Design review of the part shown in the three views and the two pictorial views. Dimensions are in mm from the part's minimum x, y and z. A direction names the side the tool comes from. Round coordinates to 2 decimals unless told otherwise and drop trailing zeros. Order: outer loops, then holes, each group sorted by start corner. A loop starts at its lowest first (then second) coordinate and runs counter-clockwise, first axis right, second up. Notation, with made-up numbers: (54.5, -11.5) - (70.5, -11.5) arc R24 ccw to (70.5, 24.5) - close; hole circle Ø8 at (1.25, -6.75). An arc over 180 degrees is marked (long way). One line per question, with ' | ' between items. Start each with the question number.
Item 1: Add section B-B on x = 28. State the section outline as (y, z) points, and give its area (3 significant figures).
Item 2: Add section C-C on y = 19. State the section outline as (x, z) points.
Item 3: Tool access review of the marked faces 1, 2 and 3: name each direction out of +Z, -Z, +X, -X, +Y, -Y from which nothing blocks a thin tool from reaching the whole face with its end or side.
Item 4: Add section A-A on z = 64. State the section outline as (x, y) points.
Item 5: For L1, parallel to Y at x = 22, z = 87.5; L2, parallel to Z at x = 46.5, y = 17; L3, parallel to X at y = 29, z = 69.5 (1 decimal), list the stretches that pass through material, from the lowest coordinate up. Write a range as [from, to].
Item 6: Add section D-D on z = 85. State the section outline as (x, y) points.
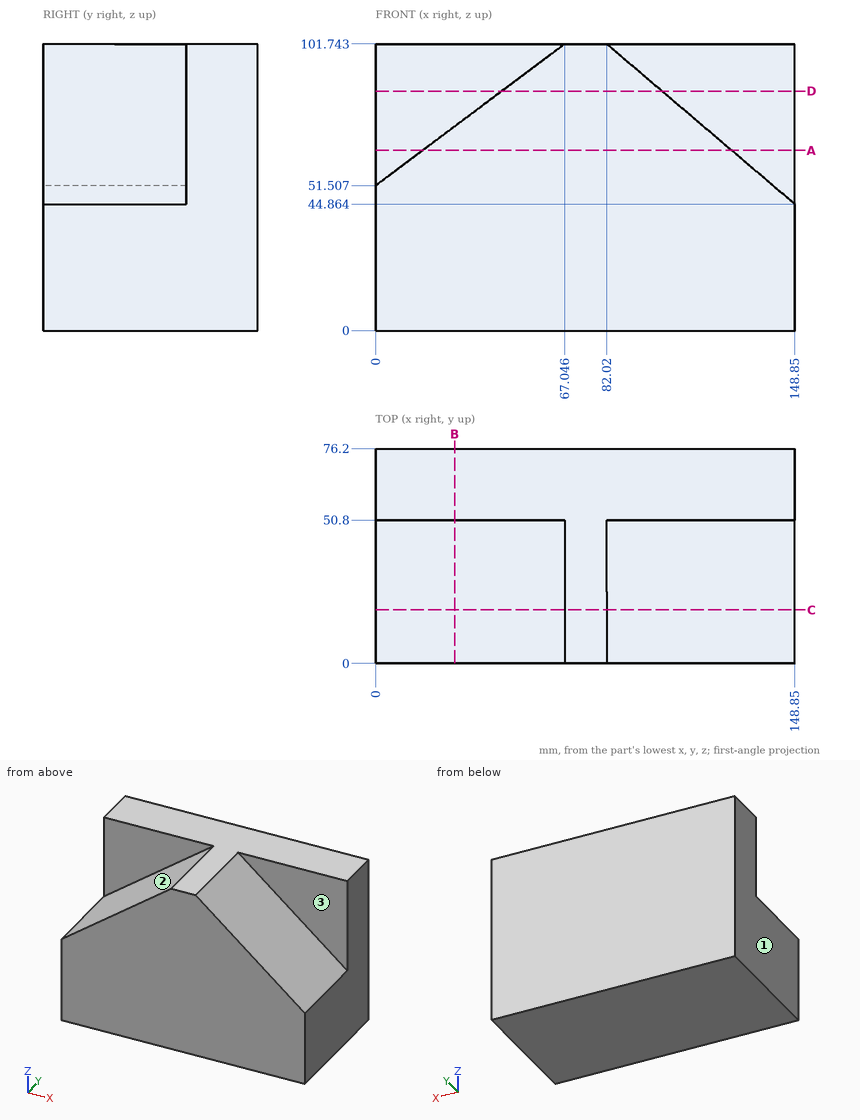
Determined:
1) outline: (0, 0) - (76.2, 0) - (76.2, 101.74) - (50.8, 101.74) - (50.8, 72.49) - (0, 72.49) - close | area: 6,270 mm2
2) outline: (0, 0) - (148.85, 0) - (148.85, 44.86) - (82.02, 101.74) - (67.05, 101.74) - (0, 51.51) - close
3) face 1: +Z, -Z, -X, +Y, -Y | face 2: +Z, -X, -Y | face 3: +Z, +X, -Y
4) outline: (0, 50.8) - (16.67, 50.8) - (16.67, 0) - (126.37, 0) - (126.37, 50.8) - (148.85, 50.8) - (148.85, 76.2) - (0, 76.2) - close
5) L1: [50.8, 76.2] | L2: [0, 86.35] | L3: [24, 119.9]
6) outline: (0, 50.8) - (44.7, 50.8) - (44.7, 0) - (101.69, 0) - (101.69, 50.8) - (148.85, 50.8) - (148.85, 76.2) - (0, 76.2) - close
